from build123d import *

# Parameters (mm, degrees)
F4_W          = 98.152165938
F4_H          = 19.5652123008
F5_DEPTH      = 25
F5_DEPTH_BACK = 25
F6_W          = 12.6501991157
F6_H          = 2


# Not quite as in the source:
# - a pattern or mirror of a feature is missing from the dataset's text; its kind, count and spacing are read off the source's solid


with BuildPart() as f1:
    # F0 (on Front) → F1 (revolve)
    with BuildSketch(Plane.XZ):
        with BuildLine():
            Line((0, -50), (0, 50))
            ThreePointArc((0, 50), (-50, 0), (0, -50))
        make_face()
    revolve(axis=Axis((0, 0, 0), (0, 0, -1)))

    # F2 (on Front) → F3 (revolve, cut)
    with BuildSketch(Plane.XZ):
        with BuildLine():
            Line((-55, 52.5), (-55, 7.5))
            ThreePointArc((-55, 7.5), (-32.5, 30), (-55, 52.5))
        make_face()
    revolve(axis=Axis((-55, 0, 30), (0, 0, -1)), mode=Mode.SUBTRACT)

    # F4 (on Front) → F5 (cut, two sides)
    with BuildSketch(Plane.XZ) as f5_sk:
        with Locations((0.7781628519, 54.7826061504)):
            Rectangle(F4_W, F4_H)
    f5 = extrude(amount=-F5_DEPTH, mode=Mode.SUBTRACT) + extrude(f5_sk.sketch, amount=F5_DEPTH_BACK, mode=Mode.SUBTRACT)

    # F5_copies: F5 across plane
    add(f5.mirror(Plane(origin=(0, 0, 0), x_dir=(-1, 0, 0), z_dir=(0, 0, -1))), mode=Mode.SUBTRACT)

    # F6 (on Front) → F7 (revolve, cut)
    with BuildSketch(Plane.XZ):
        with Locations((-54.3250995579, -0.0474521765)):
            Rectangle(F6_W, F6_H)
    revolve(axis=Axis((0, 0, 21.1794096977), (0, 0, 1)), mode=Mode.SUBTRACT)


solid = f1.part
The model under review builds one solid part; all positions refer to its coordinate system, in mm. Give positions to 0.01 mm unless a question says otherwise; leave off trailing zeros. Write each loop counter-clockwise with the first axis right and the second up, starting at its lowest first coordinate (ties: lowest second). Pieces come first, ordered by that corner, then holes. Notation, with made-up numbers: M 70.25,-13 L 82.25,-13 A22 ccw 82.25,22 Z; hole C 8.25,82 d5. An arc over 180 degrees is marked long. One line per question, with ' | ' between items. Start each with the question number.
Item 1: We need section B-B on y = -9.5. Write out the cut boundary in (x, z).
Item 2: We need section D-D on z = -9. Write out the cut boundary in (x, y), plus the area to 3 significant figures.
Item 3: We need section A-A on x = 0. Write out the cut boundary in (y, z).
Item 4: Wall thickness on line 1 (Y direction, x = -18, z = -33.5); line 2 (X direction, y = -2, z = -26); line 3 (Y direction, x = -32.5, z = -1.5): over which ranges is each line inside the solid? List them lowest first. Write a range as from..to.
Item 5: We need section C-C on x = 24. Write out the cut boundary in (y, z), plus the area to 3 significant figures.
Item 6: For pin 1 (2 mm diameter, centred on x = 35, z = -3.5, fed in from +Y); pin 2 (6 mm diameter, centred on x = -4.5, z = -14, fed in from -Y); pin 3 (1 mm diameter, centred on y = -10.5, z = -34, fed in from -X), all flat-tipped, find the tip position at first contact; note any pin that passes through.
Item 7: Draft analysis for pull direction Z (two halves, no side actions). For faces 1 (the flat face through (0, 0, 45)), 2 (the flat face through (0, 0, -45)), 3 (the cylindrical face through (-45.783, -14.418, -0.033)), state which applies: released by +Z, released by -Z, zero draft, split by the parting line, or undercut.
Results found:
1) outline: M -49.08,-1.05 A49.09 ccw -19.62,-45 L 19.62,-45 A49.09 ccw 49.08,-1.05 L 47.05,-1.05 L 47.05,0.95 L 49.08,0.95 A49.09 ccw 19.62,45 L -19.62,45 A49.09 ccw -35.07,34.35 A20.4 cw -47.87,10.89 A49.09 ccw -49.08,0.95 L -47.05,0.95 L -47.05,-1.05 Z
2) outline: C 0,0 d98.37 | area: 7,600 mm2
3) outline: M -49.99,-1.05 A50 ccw -21.79,-45 L 21.79,-45 A50 ccw 49.99,-1.05 L 48,-1.05 L 48,0.95 L 49.99,0.95 A50 ccw 21.79,45 L -21.79,45 A50 ccw -49.99,0.95 L -48,0.95 L -48,-1.05 Z
4) line 1: y = -32.46..32.46 | line 2: x = -42.66..42.66 | line 3: y = -37.97..37.97
5) outline: M -43.85,-1.05 A43.86 ccw 43.85,-1.05 L 41.57,-1.05 L 41.57,0.95 L 43.85,0.95 A43.86 ccw -43.85,0.95 L -41.57,0.95 L -41.57,-1.05 Z | area: 6,040 mm2
6) pin 1: stops at y = 36.5 | pin 2: stops at y = -48.61 | pin 3: stops at x = -35.62
7) face 1: released by +Z | face 2: released by -Z | face 3: undercut
